Verification items for the finished model (mm, model axes). Face numbers are marked on the shaded views. A direction names the side the tool comes from. Coordinates: 2 decimals unless noted, no trailing zeros. Loops run counter-clockwise (first coordinate to the right, second up) from the corner with the lowest first, then second, coordinate; pieces in that order, holes last. Notation, with made-up numbers: (79, -18) - (117, -18) arc R22 cw to (117, 0) - close; hole circle Ø2 at (87, 74). An arc over 180 degrees is marked (long way). One line per item, written item: value. Start each with the question number.
(1) Gauge pin test, flat ends, axial feed: P1, Ø7, axis at y = 3.5, z = -15.5, coming from the +X side; P2, Ø3.5, axis at y = 12.5, z = -5.5, coming from the +X side; P3, Ø10, axis at x = 25.5, z = 8, coming from the -Y side; P4, Ø1.5, axis at x = 6.5, y = -4.5, coming from the -Z side. Record the tip position at first contact, or that the pin passes through.
(2) Section check B-B (x = 37.5). Count the separate pieces of the cut face and the enclosed holes in it, plus the area to 3 significant figures.
(3) Section check C-C (y = 0). Record the boundary of the cut face in (x, z), plus the area to 3 significant figures.
(4) Draft check along Y on the marked faces 6, 7, 8 and 9. Enter one of: +Y half, -Y half, draft (parallel to the pull), parting line (faces both ways), or undercut.
(5) Thickness scan on probe 1 along Y at (x, z) = (19.5, 0); probe 2 along X at (y, z) = (3.5, 19). Record the ranges inside material, lowest first. Write a range as [from, to].
(6) Set-up check for the marked faces 1, 2, 3, 4 and 5: record each of +Z, -Z, +X, -X, +Y, -Y from which the full face is reachable in a straight line by a thin tool's end or side.
(7) Section check A-A (z = 0). Record the boundary of the cut face in (x, y), plus the area to 3 significant figures.
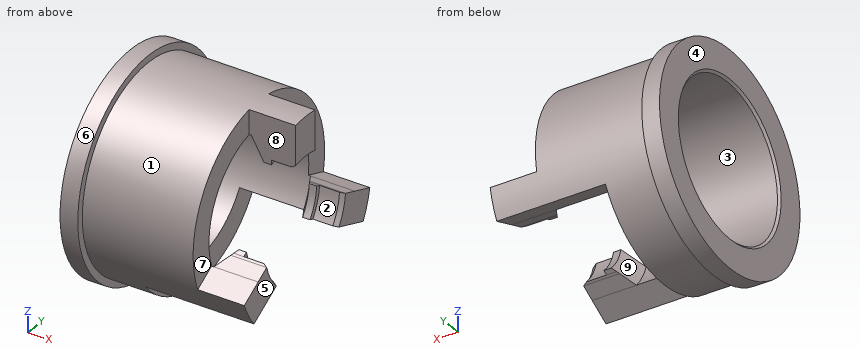
```python
from build123d import *

# Parameters (mm, degrees)
F3_DEPTH = 10.5
F4_DEPTH = 39.501
F5_DEPTH = 24.5
F6_DEPTH = 39.501


with BuildPart() as f1:
    # F0 (on Front) → F1 (revolve)
    with BuildSketch(Plane.XZ):
        Polygon((0, 24.25), (0, 17.75), (0.5, 17.25), (29.5, 17.25), (32.329016319, 12.35), (34, 12.35), (34, 13.3625), (38.5, 13.3625), (39.5, 13.9398502692), (39.5, 22.7), (4, 22.7), (4, 24.25), align=None)
    revolve(axis=Axis((21.5225653753, 0, 0), (1, 0, 0)))

    # F2 (on face) → F3 (cut)
    with BuildSketch(Plane.YZ.offset(39.5)):
        with BuildLine():
            Line((-3.35, 16.9215838502), (-3.35, 22.4514476148))
            ThreePointArc((-3.35, 22.4514476148), (-19.6587766659, 11.35), (-21.1185239862, -8.3245387047))
            Line((-21.1185239862, -8.3245387047), (-16.3295214866, -5.5596068224))
            ThreePointArc((-16.3295214866, -5.5596068224), (-14.9389382153, 8.625), (-3.35, 16.9215838502))
        make_face()
        with BuildLine():
            ThreePointArc((22.7, 0), (17.1949847339, 14.8196659881), (3.35, 22.4514476148))
            Line((3.35, 22.4514476148), (3.35, 16.9215838502))
            ThreePointArc((3.35, 16.9215838502), (14.130372764, 9.8941935271), (17.0468549562, -2.6395522541))
            Line((17.0468549562, -2.6395522541), (22.2432271297, -4.5308770514))
            ThreePointArc((22.2432271297, -4.5308770514), (22.5855181017, -2.2769216231), (22.7, 0))
        make_face()
    extrude(amount=-F3_DEPTH, mode=Mode.SUBTRACT)

    # F2 (on face) → F4 (cut, through all)
    with BuildSketch(Plane.YZ.offset(39.5)):
        with BuildLine():
            Line((-3.35, 13.5313312548), (-3.35, 16.9215838502))
            ThreePointArc((-3.35, 16.9215838502), (-14.9389382153, 8.625), (-16.3295214866, -5.5596068224))
            Line((-16.3295214866, -5.5596068224), (-13.3934766137, -3.8644805247))
            ThreePointArc((-13.3934766137, -3.8644805247), (-12.0722644581, 6.9699251346), (-3.35, 13.5313312548))
        make_face()
        with BuildLine():
            ThreePointArc((17.0468549562, -2.6395522541), (14.130372764, 9.8941935271), (3.35, 16.9215838502))
            Line((3.35, 16.9215838502), (3.35, 13.5313312548))
            ThreePointArc((3.35, 13.5313312548), (10.9776573988, 8.5913016222), (13.9398502692, 0))
            ThreePointArc((13.9398502692, 0), (13.9201386678, -0.7410566766), (13.8610596097, -1.4800175755))
            Line((13.8610596097, -1.4800175755), (17.0468549562, -2.6395522541))
        make_face()
        with BuildLine():
            Line((-3.35, 11.8869676537), (-3.35, 12.9357607527))
            ThreePointArc((-3.35, 12.9357607527), (-11.5722644581, 6.68125), (-12.8776974291, -3.5666952737))
            Line((-12.8776974291, -3.5666952737), (-11.9694159621, -3.0422987242))
            ThreePointArc((-11.9694159621, -3.0422987242), (-10.6954137367, 6.175), (-3.35, 11.8869676537))
        make_face()
        with BuildLine():
            Line((-3.35, 12.9357607527), (-3.35, 13.5313312548))
            ThreePointArc((-3.35, 13.5313312548), (-12.0722644581, 6.9699251346), (-13.3934766137, -3.8644805247))
            Line((-13.3934766137, -3.8644805247), (-12.8776974291, -3.5666952737))
            ThreePointArc((-12.8776974291, -3.5666952737), (-11.5722644581, 6.68125), (-3.35, 12.9357607527))
        make_face()
        with BuildLine():
            ThreePointArc((13.3625, 0), (10.5669480279, 8.1789984488), (3.35, 12.9357607527))
            Line((3.35, 12.9357607527), (3.35, 11.8869676537))
            ThreePointArc((3.35, 11.8869676537), (9.8461921574, 7.4548641839), (12.35, 0))
            ThreePointArc((12.35, 0), (12.3414628662, -0.4591234269), (12.3158632678, -0.917612101))
            Line((12.3158632678, -0.917612101), (13.3014064037, -1.276320467))
            ThreePointArc((13.3014064037, -1.276320467), (13.3472178621, -0.6388909066), (13.3625, 0))
        make_face()
        with BuildLine():
            ThreePointArc((13.9398502692, 0), (10.9776573988, 8.5913016222), (3.35, 13.5313312548))
            Line((3.35, 13.5313312548), (3.35, 12.9357607527))
            ThreePointArc((3.35, 12.9357607527), (10.5669480279, 8.1789984488), (13.3625, 0))
            ThreePointArc((13.3625, 0), (13.3472178621, -0.6388909066), (13.3014064037, -1.276320467))
            Line((13.3014064037, -1.276320467), (13.8610596097, -1.4800175755))
            ThreePointArc((13.8610596097, -1.4800175755), (13.9201386678, -0.7410566766), (13.9398502692, 0))
        make_face()
    extrude(amount=-F4_DEPTH, mode=Mode.SUBTRACT)

    # F2 (on face) → F5 (cut)
    with BuildSketch(Plane.YZ.offset(39.5)):
        with BuildLine():
            Line((-12.9795214866, -11.3619770278), (-17.7685239862, -14.1269089101))
            ThreePointArc((-17.7685239862, -14.1269089101), (1.9784353604, -22.6136196467), (19.9516921694, -10.8268176107))
            Line((19.9516921694, -10.8268176107), (14.7553199959, -8.9354928134))
            ThreePointArc((14.7553199959, -8.9354928134), (1.5034365624, -17.1843585421), (-12.9795214866, -11.3619770278))
        make_face()
    extrude(amount=-F5_DEPTH, mode=Mode.SUBTRACT)

    # F2 (on face) → F6 (cut, through all)
    with BuildSketch(Plane.YZ.offset(39.5)):
        with BuildLine():
            Line((-10.0434766137, -9.6668507301), (-12.9795214866, -11.3619770278))
            ThreePointArc((-12.9795214866, -11.3619770278), (1.5034365624, -17.1843585421), (14.7553199959, -8.9354928134))
            Line((14.7553199959, -8.9354928134), (11.5695246494, -7.7759581348))
            ThreePointArc((11.5695246494, -7.7759581348), (1.214938004, -13.8868049304), (-10.0434766137, -9.6668507301))
        make_face()
        with BuildLine():
            Line((-8.6194159621, -8.8446689295), (-9.5276974291, -9.369065479))
            ThreePointArc((-9.5276974291, -9.369065479), (1.1646186125, -13.3116516533), (11.0098714434, -7.5722610263))
            Line((11.0098714434, -7.5722610263), (10.0243283076, -7.2135526603))
            ThreePointArc((10.0243283076, -7.2135526603), (1.0763734229, -12.3030045214), (-8.6194159621, -8.8446689295))
        make_face()
        with BuildLine():
            Line((-9.5276974291, -9.369065479), (-10.0434766137, -9.6668507301))
            ThreePointArc((-10.0434766137, -9.6668507301), (1.214938004, -13.8868049304), (11.5695246494, -7.7759581348))
            Line((11.5695246494, -7.7759581348), (11.0098714434, -7.5722610263))
            ThreePointArc((11.0098714434, -7.5722610263), (1.1646186125, -13.3116516533), (-9.5276974291, -9.369065479))
        make_face()
    extrude(amount=-F6_DEPTH, mode=Mode.SUBTRACT)


solid = f1.part
```
Responses:
1. P1: stops at x = 15
1. P2: stops at x = 39.5
1. P3: stops at y = -22.5
1. P4: stops at z = -22.39
2. separate pieces: 3
2. enclosed holes: 0
2. area: 189 mm²
3. outline: (0, -24.25) - (4, -24.25) - (4, -22.7) - (15, -22.7) - (15, -17.25) - (0.5, -17.25) - (0, -17.75) - close; (0, 17.75) - (0.5, 17.25) - (29.5, 17.25) - (32.33, 12.35) - (34, 12.35) - (34, 13.36) - (38.5, 13.36) - (39.5, 13.94) - (39.5, 22.7) - (4, 22.7) - (4, 24.25) - (0, 24.25) - close
3. area: 345 mm²
4. face 6: parting line
4. face 7: draft
4. face 8: -Y half
4. face 9: undercut
5. probe 1: y = [-22.7, -17.25], [17.25, 22.7]
5. probe 2: x = [0, 29]
6. face 1: +X
6. face 2: +Z, +X
6. face 3: -X
6. face 4: +Z, -Z, -X, +Y, -Y
6. face 5: +Z, -Z, +X, +Y, -Y
7. outline: (0, -24.25) - (4, -24.25) - (4, -22.7) - (29, -22.7) - (29, -17.25) - (0.5, -17.25) - (0, -17.75) - close; (0, 17.75) - (0.5, 17.25) - (29, 17.25) - (29, 22.7) - (4, 22.7) - (4, 24.25) - (0, 24.25) - close
7. area: 328 mm²
